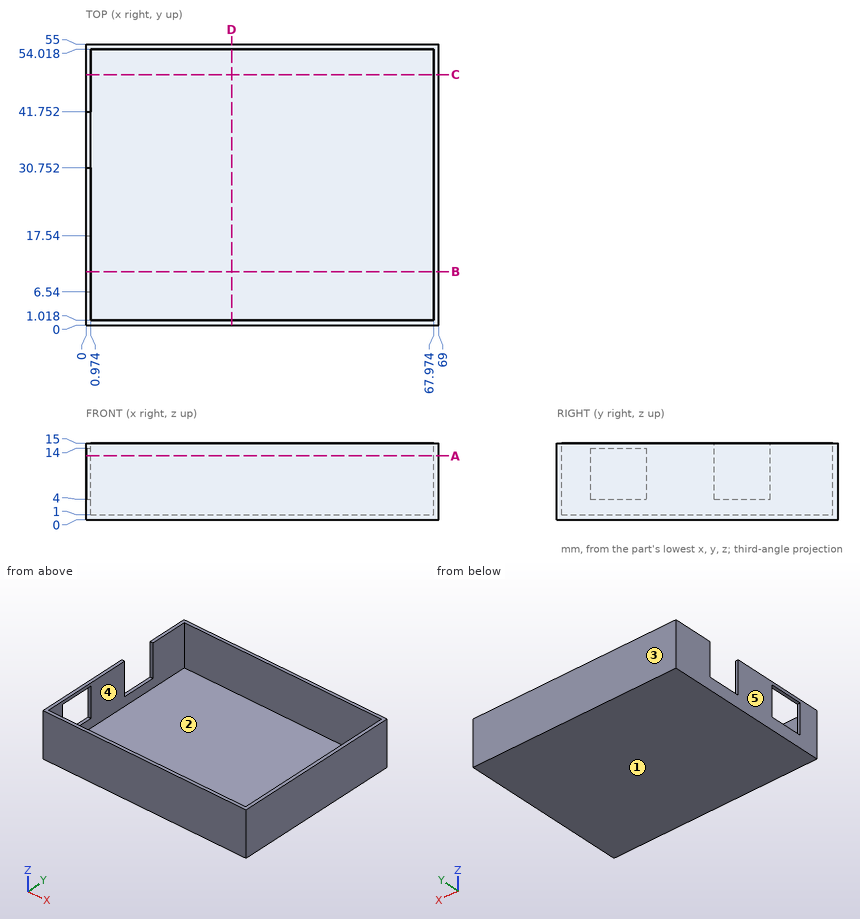
Can you work these out from the drawing? Everything is in mm from the part's minimum corner. A direction names the side the tool comes from. Give positions to 0.01 mm unless a question says otherwise; leave off trailing zeros. Order: outer loops, then holes, each group sorted by start corner. A loop starts at its lowest first (then second) coordinate and runs counter-clockwise, first axis right, second up. Notation, with made-up numbers: M 54,82.5 L 88,82.5 A19 ccw 88,113.5 Z; hole C 42.25,-21 d9. An arc over 180 degrees is marked long. Use a Markdown table: item, result. Add a question column.
1. On a 3-axis mill with a long thin cutter (end or side, diameter ignored), from which of +Z, -Z, +X, -X, +Y, -Y can I reach the whole of each face in a straight line? I mean the marked faces 1 and 2. Say none if no direction works.
2. Suppose I cut it at C-C (y = 49). List the corners of the cut face in (x, z) for me (1 decimal).
3. For pin 1 Ø4 at (y, z) = (37.5, 8.5) entering from -X; pin 2 Ø0.8 at (x, y) = (0.5, 37) entering from +Z; pin 3 Ø16 at (x, y) = (27, 40.5) entering from +Z, each with a flat end and sliding along its axis, tell me the tip position at first contact or that it passes through.
4. If we mould it in two halves opening along X, with no side actions, what happens to the marked faces 3, 4 and 5? For each: +X half, -X half, draft (parallel to the pull), parting line (faces both ways), or undercut.
5. Suppose I cut it at D-D (x = 28.5). List the corners of the cut face in (y, z) for me.
6. I need wall thicknesses on probe 1 along Y at (x, z) = (47.5, 9.5); probe 2 along X at (y, z) = (48.5, 1.25) (1 decimal); probe 3 along X at (y, z) = (40, 6) (1 decimal). Which ranges of each line are inside material? Lowest first, please. Write a range as from..to.
7. Suppose I cut it at B-B (y = 10.5). List the corners of the cut face in (x, z) for me (1 decimal).
8. Suppose I cut it at A-A (z = 12.5). List the corners of the cut face in (x, y) for me (1 decimal).
Results list:
| question | item | result |
|---|---|---|
| 1 | face 1 | -Z, +X, -X, +Y, -Y |
| 1 | face 2 | +Z |
| 2 | outline | M 0,0 L 69,0 L 69,15 L 68,15 L 68,1 L 1,1 L 1,15 L 0,15 Z |
| 3 | pin 1 | stops at x = 67.97 |
| 3 | pin 2 | stops at z = 4 |
| 3 | pin 3 | stops at z = 1 |
| 4 | face 3 | draft |
| 4 | face 4 | undercut |
| 4 | face 5 | -X half |
| 5 | outline | M 0,0 L 55,0 L 55,15 L 54.02,15 L 54.02,1 L 1.02,1 L 1.02,15 L 0,15 Z |
| 6 | probe 1 | y = 0..1.02, 54.02..55 |
| 6 | probe 2 | x = 0..1, 68..69 |
| 6 | probe 3 | x = 68..69 |
| 7 | outline | M 0,0 L 69,0 L 69,15 L 68,15 L 68,1 L 1,1 L 1,4 L 0,4 Z; M 0,14 L 1,14 L 1,15 L 0,15 Z |
| 8 | outline | M 0,0 L 69,0 L 69,55 L 0,55 L 0,41.8 L 1,41.8 L 1,54 L 68,54 L 68,1 L 1,1 L 1,6.5 L 0,6.5 Z; M 0,17.5 L 1,17.5 L 1,30.8 L 0,30.8 Z |
